Autodesk Inventor part; units mm, degrees
ref_plane "YZ Plane" through (0, 0, 0) normal (1, 0, 0) x (0, 1, 0)
ref_plane "XZ Plane" through (0, 0, 0) normal (0, 1, 0) x (-1, 0, 0)
ref_plane "XY Plane" through (0, 0, 0) normal (0, 0, 1) x (1, 0, 0)
sketch "Sketch1" plane through (0, 0, 0) normal (0, 0, 1) x (1, 0, 0)
  line L0 (0, 0) -> (0, 10)
  line L1 (0, 10) -> (4.6, 10)
  line L2 (4.6, 10) -> (4.6, 2.5)
  line L3 (4.6, 2.5) -> (7.6, 2.5)
  line L4 (7.6, 2.5) -> (7.6, 10)
  line L5 (7.6, 10) -> (12.2, 10)
  line L6 (12.2, 10) -> (12.2, 0)
  line L7 (12.2, 0) -> (0, 0)
  dimension "d0" = 12.2
  dimension "d1" = 10
  dimension "d2" = 7.5
  dimension "d3" = 3
extrude "Extrusion1" add sketch "Sketch1" along normal blind 5
sketch "Sketch2" plane through (0, 0, 0) normal (0, -1, 0) x (1, 0, 0)
  line L0 (0, 0) -> (0, 5)
  line L1 (1.5, 3.77) -> (10.7, 3.77) construction
  line L2 (0, 5) -> (12.2, 5) construction
  line L3 (1.275, 3.995) -> (1.725, 3.995)
  line L4 (1.725, 3.995) -> (1.725, 3.545)
  line L5 (1.725, 3.545) -> (1.275, 3.545)
  line L6 (1.275, 3.545) -> (1.275, 3.995)
  line L7 (1.275, 3.995) -> (1.725, 3.545) construction
  line L8 (1.725, 3.995) -> (1.275, 3.545) construction
  point P0 (1.5, 1.23)
  point P1 (3, 2.5)
  point P2 (10.7, 1.23)
  point P3 (0, 2.5)
  point P4 (6.1, 3.77)
  point P5 (6.1, 5)
  dimension "d6" = 1.27
  dimension "d7" = 1.27
  dimension "d8" = 1.5
  dimension "d9" = 9.2
  dimension "d10" = 0.45
  dimension "d11" = 0.45
extrude "Extrusion2" add sketch "Sketch2" along normal blind 9
pattern_sketch "Sketch Driven Pattern1" of "Extrusion2" from (1.5, 0, 3.77) copies at (1.5, 0, 1.23) at (3, 0, 2.5) at (10.7, 0, 3.77) at (10.7, 0, 1.23)
chamfer "Chamfer1" distance 0.75 angle 45 2 edges at (9.9, 10, 0) (2.3, 10, 0)
properties part number "GP1A52HRJ00F (Large slot detector)"
Could you check a few things on this model? Use its own coordinates, in mm. A direction names the side the tool comes from. Give positions to 0.01 mm unless a question says otherwise; leave off trailing zeros. Write each loop counter-clockwise with the first axis right and the second up, starting at its lowest first coordinate (ties: lowest second). Pieces come first, ordered by that corner, then holes. Notation, with made-up numbers: (-8.5, 18.25) - (2.5, 18.25) arc R26 cw to (2.5, 34.25) - close; hole circle Ø2 at (-8, 5). An arc over 180 degrees is marked (long way). One line per item, written item: value. Start each with the question number.
Item 1: Please list where these lines run through material, in increasing order: line 1 (X direction, y = 4.25, z = 4.65); line 2 (X direction, y = -4.5, z = 3.9) (3 decimals); line 3 (Y direction, x = 5.75, z = 3.7). Write a range as from..to.
Item 2: Which directions (+Z, -Z, +X, -X, +Y, -Y) give clear straight access to the entire face, cutting with the end or side of a thin tool? Please do faces 1 (the face through (2, 10, 3)), 2 (the face through (7.6, 6, 2)).
Item 3: Imagine slicing it at C-C, the plane x = 10. List the corners of the cut face in (y, z) for me, and give its area (3 significant figures).
Item 4: I'm going to push flat-ended pins straight in: pin 1 (0.5 mm diameter, centred on y = -6.5, z = 2.5, fed in from +X) (3 decimals); pin 2 (0.5 mm diameter, centred on y = -6, z = 4, fed in from +X) (3 decimals); pin 3 (0.5 mm diameter, centred on x = 1.5, y = -6, fed in from -Z) (3 decimals). Where does each tip first touch, or does it pass through?
Item 5: Imagine slicing it at D-D, the plane z = 1.65. List the corners of the cut face in (x, y) for me, and give its area (3 significant figures).
Item 6: Imagine slicing it at B-B, the plane y = -3.25. List the corners of the cut face in (x, z) for me (3 decimals).
Item 7: Imagine slicing it at A-A, the plane y = 8.25. List the corners of the cut face in (x, z) for me, and give its area (3 significant figures).
Geometry says:
1. line 1: 0..4.6, 7.6..12.2
1. line 2: 1.275..1.725, 10.475..10.925
1. line 3: 0..2.5
2. face 1: +Z, -Z, +X, -X, +Y
2. face 2: +Z, -Z, +Y
3. outline: (0, 0) - (9.25, 0) - (10, 0.75) - (10, 5) - (0, 5) - close
3. area: 49.7 mm^2
4. pin 1: x = 3.225
4. pin 2: x = 10.925
4. pin 3: z = 1.005
5. outline: (0, 0) - (12.2, 0) - (12.2, 10) - (7.6, 10) - (7.6, 2.5) - (4.6, 2.5) - (4.6, 10) - (0, 10) - close
5. area: 99.5 mm^2
6. outline: (1.275, 1.005) - (1.725, 1.005) - (1.725, 1.455) - (1.275, 1.455) - close; (1.275, 3.545) - (1.725, 3.545) - (1.725, 3.995) - (1.275, 3.995) - close; (2.775, 2.275) - (3.225, 2.275) - (3.225, 2.725) - (2.775, 2.725) - close; (10.475, 1.005) - (10.925, 1.005) - (10.925, 1.455) - (10.475, 1.455) - close; (10.475, 3.545) - (10.925, 3.545) - (10.925, 3.995) - (10.475, 3.995) - close
7. outline: (0, 0) - (4.6, 0) - (4.6, 5) - (0, 5) - close; (7.6, 0) - (12.2, 0) - (12.2, 5) - (7.6, 5) - close
7. area: 46.0 mm^2
